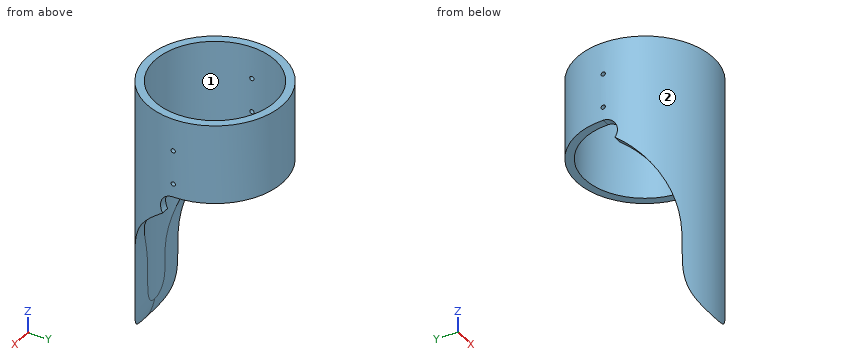
```python
from build123d import *

# Parameters (mm, degrees)
SKETCH1_R               = 50.875
SKETCH1_R_2             = 44.875
BOSS_EXTRUDE1_DEPTH     = 258
SKETCH2_OUTSIDE_W       = 319.084
SKETCH2_OUTSIDE_H       = 162.834
CUT_EXTRUDE1_DEPTH      = 51.875
CUT_EXTRUDE1_DEPTH_BACK = 51.875
SKETCH4_R               = 1.5875
CUT_EXTRUDE3_DEPTH      = 51.8750001
CUT_EXTRUDE3_DEPTH_BACK = 51.8750001


with BuildPart() as part:
    # Sketch1 → Boss-Extrude1 (new body)
    with BuildSketch(Plane.XY):
        Circle(SKETCH1_R)
        Circle(SKETCH1_R_2, mode=Mode.SUBTRACT)
    extrude(amount=BOSS_EXTRUDE1_DEPTH)

    # Sketch2 outside → Cut-Extrude1 (cut, two sides)
    with BuildSketch(Plane(origin=(0, 0, 0), x_dir=(0, 0, -1), z_dir=(1, 0, 0))) as cut_extrude1_sk:
        with Locations((-129, 0)):
            Rectangle(SKETCH2_OUTSIDE_W, SKETCH2_OUTSIDE_H)
        with BuildLine():
            Line((-198.5, -50.875), (0, -50.875))
            add(Edge.make_bspline(
                [(-123.386550588, -8.275819337), (-81.752620628, -64.643145872), (-28.413904024, -31.213109934), (0, -50.875)],
                knots=[0.043569277, 0.043569277, 0.043569277, 0.043569277, 1, 1, 1, 1], degree=3))
            ThreePointArc((-123.386550588, -8.275819337), (-133.683241713, -8.835567161), (-139, 0))
            Line((-139, 0), (-139, 50.875))
            Line((-139, 50.875), (-198.5, 50.875))
            Line((-198.5, 50.875), (-198.5, -50.875))
        make_face(mode=Mode.SUBTRACT)
    extrude(amount=CUT_EXTRUDE1_DEPTH, mode=Mode.SUBTRACT)
    extrude(cut_extrude1_sk.sketch, amount=-CUT_EXTRUDE1_DEPTH_BACK, mode=Mode.SUBTRACT)

    # Sketch4 → Cut-Extrude3 (cut, two sides)
    with BuildSketch(Plane(origin=(0, 0, 0), x_dir=(0, 0, -1), z_dir=(1, 0, 0))) as cut_extrude3_sk:
        with Locations((-149, 0)):
            Circle(SKETCH4_R)
        with Locations((-174.4, 0)):
            Circle(SKETCH4_R)
    extrude(amount=CUT_EXTRUDE3_DEPTH, mode=Mode.SUBTRACT)
    extrude(cut_extrude3_sk.sketch, amount=-CUT_EXTRUDE3_DEPTH_BACK, mode=Mode.SUBTRACT)


solid = part.part
```
Geometry check sheet. Reference: the model listing, model coordinates, mm. Face numbers are marked on the shaded views. Round coordinates to 2 decimals unless told otherwise and drop trailing zeros. Order: outer loops, then holes, each group sorted by start corner. A loop starts at its lowest first (then second) coordinate and runs counter-clockwise, first axis right, second up. Notation, with made-up numbers: (-18.5, 32.25) - (-11.5, 32.25) arc R27 cw to (-11.5, 55.25) - close; hole circle Ø11 at (-36, -9). An arc over 180 degrees is marked (long way). Use a Markdown table: item, result. Add a question column.
(1) Sectioned sample at A-A, the plane y = 15. Enter the section's corners in (x, z).
(2) Depth check by flat-ended pin: pin 1 (10 mm diameter, centred on x = -17, y = -31, fed in from -Z); pin 2 (10 mm diameter, centred on y = -40, z = 143, fed in from -X); pin 3 (8 mm diameter, centred on x = -16, z = 119.5, fed in from +Y); pin 4 (12 mm diameter, centred on x = -32.5, z = 109.5, fed in from -Y). Enter the tip coordinate at first touch or a pass-through.
(3) Sectioned sample at B-B, the plane y = 34. Enter the section's corners in (x, z).
(4) Release check for a two-part mould opening along X. For the marked faces 1 and 2 record: pulls with the +X half, pulls with the -X half, needs draft (parallel to the pull), parting line crosses it, or undercut.
(5) Material ranges on line 1 along Z through (x, y) = (47, 0); line 2 along X through (y, z) = (-1, 156.5); line 3 along X through (y, z) = (-33.5, 149.5), recorded low to high. Write a range as [from, to].
Answers below:
| question | item | result |
|---|---|---|
| 1 | outline | (-48.61, 139) - (-42.29, 139) - (-42.29, 198.5) - (-48.61, 198.5) - close; (42.29, 139) - (48.61, 139) - (48.61, 198.5) - (42.29, 198.5) - close |
| 2 | pin 1 | through |
| 2 | pin 2 | x = -36.92 |
| 2 | pin 3 | y = -40.17 |
| 2 | pin 4 | y = -43.43 |
| 3 | outline | (-37.85, 139) - (-29.29, 139) - (-29.29, 198.5) - (-37.85, 198.5) - close; (29.29, 139) - (37.85, 139) - (37.85, 198.5) - (29.29, 198.5) - close |
| 4 | face 1 | undercut |
| 4 | face 2 | parting line crosses it |
| 5 | line 1 | [139, 147.41], [150.59, 172.81], [175.99, 198.5] |
| 5 | line 2 | [-50.87, -44.86], [44.86, 50.87] |
| 5 | line 3 | [-38.29, -29.86], [29.86, 38.29] |
